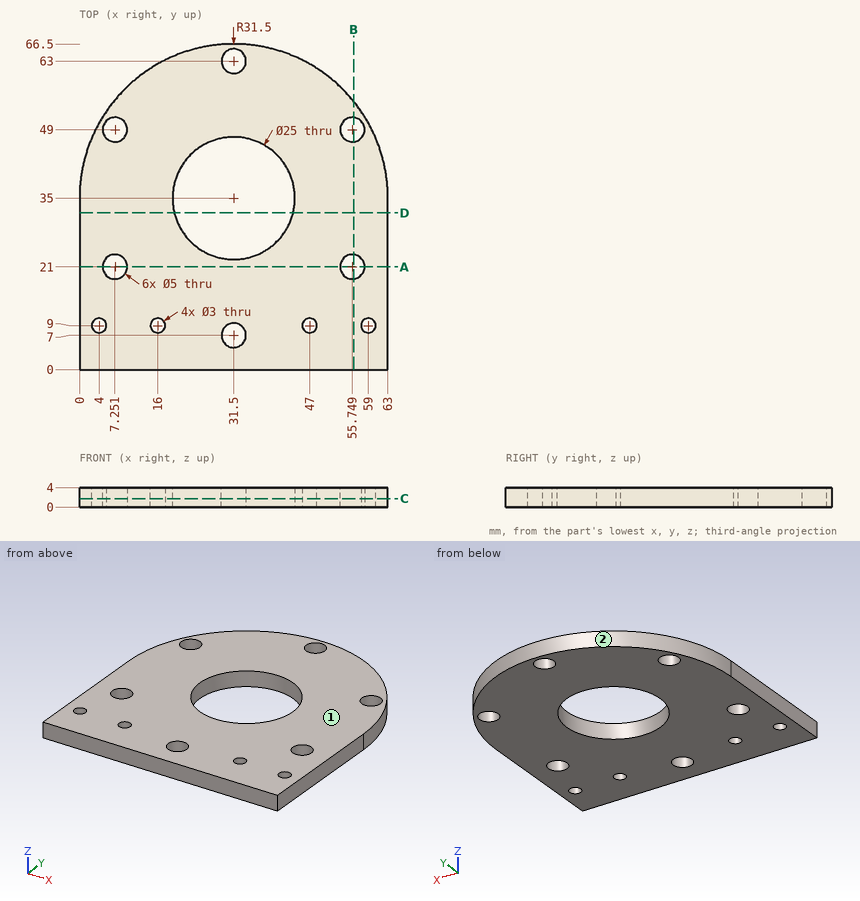
Input: dimensioned drawing with shaded views. Units: mm. Origin: part minimum x, y, z. Give positions to 0.01 mm unless a question says otherwise; leave off trailing zeros. Write each loop counter-clockwise with the first axis right and the second up, starting at its lowest first coordinate (ties: lowest second). Pieces come first, ordered by that corner, then holes.
Q1. Pull-direction query (Y, two-part tool) for the marked faces 1 and 2; classes: pulls with the +Y half, pulls with the -Y half, needs draft (parallel to the pull), parting line crosses it, or undercut.
Q2. Section C-C, the plane z = 1.75. State how many separate pieces and enclosed holes the cut face has, plus the area to 3 significant figures.
Q3. First-contact query: P1, Ø8, axis at x = 55.75, y = 49, coming from the -Z side; P2, Ø1, axis at y = 48.5, z = 1.5, coming from the +X side. Flat tips, straight axial feed; report the tip coordinate or a pass-through.
Q4. Section A-A, the plane y = 21. Output: boundary loops of the cut face in (x, z), plus the area to 3 significant figures.
Q5. Material intervals for probe 1 along Y at (x, z) = (31.5, 1.8); probe 2 along Y at (x, z) = (54, 3.3) (1 decimal); probe 3 along Y at (x, z) = (58, 1) (1 decimal), sorted ascending.
Q6. Section D-D, the plane y = 32. Output: boundary loops of the cut face in (x, z) (1 decimal).
Q7. Section B-B, the plane x = 56. Output: boundary loops of the cut face in (y, z), plus the area to 3 significant figures.
Filled in:
1. face 1: needs draft
1. face 2: pulls with the +Y half
2. separate pieces: 1
2. enclosed holes: 11
2. area: 3,130 mm2
3. P1: stops at z = 0
3. P2: stops at x = 60.19
4. outline: (0, 0) - (4.75, 0) - (4.75, 4) - (0, 4) - close; (9.75, 0) - (53.25, 0) - (53.25, 4) - (9.75, 4) - close; (58.25, 0) - (63, 0) - (63, 4) - (58.25, 4) - close
4. area: 212 mm2
5. probe 1: y = 0 to 4.5, 9.5 to 22.5, 47.5 to 60.5, 65.5 to 66.5
5. probe 2: y = 0 to 19.2, 22.8 to 47.2, 50.8 to 57
5. probe 3: y = 0 to 7.9, 10.1 to 19.9, 22.1 to 47.9, 50.1 to 52
6. outline: (0, 0) - (19.4, 0) - (19.4, 4) - (0, 4) - close; (43.6, 0) - (63, 0) - (63, 4) - (43.6, 4) - close
7. outline: (0, 0) - (18.51, 0) - (18.51, 4) - (0, 4) - close; (23.49, 0) - (46.51, 0) - (46.51, 4) - (23.49, 4) - close; (51.49, 0) - (54.8, 0) - (54.8, 4) - (51.49, 4) - close
7. area: 179 mm2
